Source: CAD feature listing. Evaluate the final solid. Frame: model axes, mm. A direction names the side the tool comes from. Coordinates: 2 decimals unless noted, no trailing zeros. Order: outer loops, then holes, each group sorted by start corner. A loop starts at its lowest first (then second) coordinate and runs counter-clockwise, first axis right, second up. Notation, with made-up numbers: (39.5, 74) -> (44.5, 74) arc R23 ccw to (44.5, 99) -> close; hole circle Ø4 at (84.25, -20). An arc over 180 degrees is marked (long way). Put each result on its own line as item: value.
Autodesk Inventor part; units mm, degrees
ref_plane "YZ Plane" through (0, 0, 0) normal (1, 0, 0) x (0, 1, 0)
ref_plane "XZ Plane" through (0, 0, 0) normal (0, 1, 0) x (-1, 0, 0)
ref_plane "XY Plane" through (0, 0, 0) normal (0, 0, 1) x (1, 0, 0)
sketch "Sketch1" plane through (0, 0, 0) normal (0, 1, 0) x (-1, 0, 0)
  line L0 (20, 0) -> (0, 0)
  line L1 (0, 0) -> (0, -57.5)
  line L2 (0, -57.5) -> (20, -57.5)
  line L3 (20, -57.5) -> (20, 0)
  circle A0 centre (10, -7.75) radius 2.5
  circle A1 centre (10, -25.75) radius 2.5
  circle A2 centre (10, -43.75) radius 2.5
  line L4 (15, -54.25) -> (5, -54.25)
  line L5 (5, -54.25) -> (5, -56.75)
  line L6 (5, -56.75) -> (15, -56.75)
  line L7 (15, -56.75) -> (15, -54.25)
  circle A3 centre (10, -7.75) radius 3
  circle A4 centre (10, -25.75) radius 3
  circle A5 centre (10, -43.75) radius 3
  dimension "d0" = 57.5
  dimension "d1" = 20
  dimension "d2" = 5
  dimension "d3" = 5
  dimension "d4" = 5
  dimension "d8" = 0.75
  dimension "d9" = 2.5
  dimension "d10" = 10
  dimension "d20" = 10
  dimension "d21" = 5
  dimension "d22" = 6
  dimension "d23" = 6
  dimension "d24" = 6
  dimension "d45" = 7.75
  dimension "d46" = 18
  dimension "d47" = 18
extrude "Extrusion1" add sketch "Sketch1" against normal blind 1.4 contours L3 L2 L1 L0 | A0 | A1 | A2 | L7 L6 L5 L4 | A3 | A4 | A5
extrude "Extrusion2" add sketch "Sketch1" along normal blind 12 contours L7 L6 L5 L4
extrude "Extrusion5" add sketch "Sketch1" along normal blind 8 contours A0
extrude "Extrusion6" add sketch "Sketch1" along normal blind 1 contours A3
fillet "Fillet4" radius 2.5 1 edges at (-7.5, 8, -7.75)
extrude "Extrusion7" add sketch "Sketch1" along normal blind 1 contours A4
extrude "Extrusion8" add sketch "Sketch1" along normal blind 8 contours A1
fillet "Fillet5" [suppressed]
extrude "Extrusion9" add sketch "Sketch1" along normal blind 8 contours A2
extrude "Extrusion10" add sketch "Sketch1" along normal blind 1 contours A5
fillet "Fillet6" radius 2.5 1 edges at (-7.5, 8, -43.75)
sketch "Sketch2" plane through (-10, 8, -25.75) normal (0, 1, 0) x (1, 0, 0)
  point P0 (10, -25.75)
  point P1 (0, 0)
properties part number "Led_Board_V1"
1. Pull-direction query (Z, two-part tool) for faces 5 (the flat face through (-10, -1, -57.5)), 6 (the flat face through (-5, 6, -55)), 7 (the cylindrical face through (-11.61, 0.49, -10.28)); classes: pulls with the +Z half, pulls with the -Z half, needs draft (parallel to the pull), parting line crosses it, or undercut.
Numbers:
face 5: pulls with the -Z half
face 6: needs draft
face 7: undercut
2. Ray query, line 1 along Z through (x, y) = (-10, 3.5); line 2 along Z through (x, y) = (-9.75, 0.5); line 3 along X through (y, z) = (1.5, -44). Return the intervals inside material, ascending.
Numbers:
line 1: z = -56.75 to -54.25, -46.25 to -41.25, -28.25 to -23.25, -10.25 to -5.25
line 2: z = -56.75 to -54.25, -46.74 to -40.76, -28.74 to -22.76, -10.74 to -4.76
line 3: x = -12.49 to -7.51
3. Cut plane C-C on z = -25.75. Output: boundary loops of the cut face in (x, y).
Numbers:
outline: (-20, -1.4) -> (0, -1.4) -> (0, 0) -> (-7, 0) -> (-7, 1) -> (-7.5, 1) -> (-7.5, 8) -> (-12.5, 8) -> (-12.5, 1) -> (-13, 1) -> (-13, 0) -> (-20, 0) -> close
4. Set-up query: faces 1 (the flat face through (-10, 6, -56.75)), 2 (the flat face through (-10, 8, -26)), 3 (the flat face through (-15, 6, -56)), 4 (the cylindrical face through (-12.77, 0.49, -24.6)). Return all of +Z, -Z, +X, -X, +Y, -Y with unobstructed straight access to the full face (end or side cutting, diameter ignored); none if empty.
Numbers:
face 1: -Z, +X, -X, +Y
face 2: +Z, +X, -X, +Y
face 3: +Z, -Z, -X, +Y
face 4: +Y
5. Cut plane A-A on y = 7. Output: boundary loops of the cut face in (x, z), plus the area to 3 significant figures.
Numbers:
outline: (-15, -56.75) -> (-5, -56.75) -> (-5, -54.25) -> (-15, -54.25) -> close; circle Ø5 at (-10, -25.75); circle Ø4 at (-10, -43.75); circle Ø4 at (-10, -7.75)
area: 69.8 mm2
6. Cut plane D-D on z = -7.75. Output: boundary loops of the cut face in (x, y), plus the area to 3 significant figures.
Numbers:
outline: (-20, -1.4) -> (0, -1.4) -> (0, 0) -> (-7, 0) -> (-7, 1) -> (-7.5, 1) -> (-7.5, 5.5) arc R2.5 ccw to (-12.5, 5.5) -> (-12.5, 1) -> (-13, 1) -> (-13, 0) -> (-20, 0) -> close
area: 66.3 mm2
7. First-contact query: pin 1 (3 mm diameter, centred on x = -12, y = 7, fed in from -Z); pin 2 (1.8 mm diameter, centred on x = -9, z = -24.5, fed in from +Y); pin 3 (1.2 mm diameter, centred on y = 6.5, z = -56, fed in from +X). Flat tips, straight axial feed; report the tip coordinate or a pass-through.
Numbers:
pin 1: stops at z = -56.75
pin 2: stops at y = 8
pin 3: stops at x = -5
